Model file for the job. Use its own axes, mm. A direction names the side the tool comes from. Round coordinates to 2 decimals unless told otherwise and drop trailing zeros. Loops run counter-clockwise (first coordinate to the right, second up) from the corner with the lowest first, then second, coordinate; pieces in that order, holes last. Notation, with made-up numbers: M -14.75,27 L -3.75,27 A26 cw -3.75,65 Z; hole C 11.25,62.5 d11. An arc over 180 degrees is marked long. Use a Markdown table: item, result. Add a question column.
Q1. Cut at A-A (y = 0). Give the cut face in (x, z), plus the area to 3 significant figures.
Q2. Pin check, flat tips, straight feed: pin 1 (2.5 mm diameter, centred on y = 0, z = 2.5, fed in from +X); pin 2 (6.5 mm diameter, centred on x = 0, y = 0, fed in from +Z); pin 3 (1 mm diameter, centred on y = 6, z = 1.5, fed in from -X); pin 4 (3 mm diameter, centred on x = 3, z = 1.5, fed in from +Y). Stop position of each tip, or through.
Q3. Mould opens along Y. For faces 1 (the face through (-2.37, 4.495, 3.987)), 2 (the face through (3.81, -6.46, 2.46)), 3 (the face through (7.6, 2.5, 2.5)) say: +Y half, -Y half, draft (parallel to the pull), parting line (faces both ways), or undercut.
Q4. Probe line 1 (Z direction, x = 6.25, y = 0); line 2 (Y direction, x = 0, z = 1.95); line 3 (X direction, y = 0, z = 1.35). List the from-to ranges inside material, lowest first. Write a range as from..to.
Q5. Tool access for faces 4 (the face through (-5.947, 5.301, 2.465)), 5 (the face through (5, 0, 4)), 6 (the face through (8.071, -1, 1)), 7 (the face through (7.6, -2.5, 2.5)): list every direction of +Z, -Z, +X, -X, +Y, -Y with a clear straight run to the whole face (end or side of a thin tool).
Q6. Cut at C-C (x = 3.5). Give the cut face in (y, z).
Q7. Cut at D-D (x = 1.5). Give the cut face in (y, z).
Q8. Cut at B-B (z = 2.5). Give the cut face in (x, y), plus the area to 3 significant figures.
Autodesk Fusion 360 part; units mm, degrees
sketch "Boceto1" plane through (0, 0, 0) normal (0, 0, 1) x (1, 0, 0)
  circle A0 centre (0, 0) radius 2.5
  circle A1 centre (0, 0) radius 7.5
  line L0 (0, 2.5) -> (7.0711, 2.5)
  line L1 (0, -2.5) -> (7.0711, -2.5)
  line L2 (7.0711, 2.5) -> (7.0711, -2.5)
  line L3 (7.0711, 2.5) -> (8.0711, 2.5)
  line L4 (8.0711, 2.5) -> (8.0711, -2.5)
  line L5 (8.0711, -2.5) -> (7.0711, -2.5)
  line L6 (-6.2006, 5.7397) -> (-1.8705, 8.2397)
  line L7 (-5.7006, 4.8737) -> (-6.2006, 5.7397)
  line L8 (-1.8705, 8.2397) -> (-1.3705, 7.3737)
  line L9 (-1.8705, -8.2397) -> (-6.2006, -5.7397)
  line L10 (-1.3705, -7.3737) -> (-1.8705, -8.2397)
  line L11 (-6.2006, -5.7397) -> (-5.7006, -4.8737)
  dimension "d1" = 5
  dimension "d2" = 15
  dimension "d3" = 1
  dimension "d5" = 360
extrude "Extruir1" add sketch "Boceto1" along normal blind 5 contours A0 L0 L1 L2 | A0 A1 L0 L1 | A1 L3 L4 L5 | A1 L2 | A1 L6 L7 L8 | A1 L9 L10 L11
sketch "Boceto2" plane through (-4.0355, -6.9897, 0) normal (-0.5, -0.866, 0) x (0.866, -0.5, 0)
  line L0 (-2.5, 0) -> (2.5, 0)
  line L1 (2.5, 0) -> (2.5, 5)
  line L2 (2.5, 5) -> (-2.5, 5)
  line L3 (-2.5, 5) -> (-2.5, 0)
  line L4 (-2.5, 5) -> (2.5, 0)
  line L5 (2.5, 5) -> (-2.5, 0)
  circle A0 centre (0, 2.5) radius 1.5
  dimension "d8" = 3
sketch "Boceto3" plane through (8.0711, 0, 0) normal (1, 0, 0) x (0, 1, 0)
  line L0 (-2.5, 0) -> (2.5, 0)
  line L1 (2.5, 0) -> (2.5, 5)
  line L2 (2.5, 5) -> (-2.5, 5)
  line L3 (-2.5, 5) -> (-2.5, 0)
  line L4 (-2.5, 5) -> (2.5, 0)
  line L5 (2.5, 5) -> (-2.5, 0)
  circle A0 centre (0, 2.5) radius 1.5
  dimension "d9" = 3
sketch "Boceto4" plane through (-4.0355, 6.9897, 0) normal (-0.5, 0.866, 0) x (-0.866, -0.5, 0)
  line L0 (-2.5, 0) -> (2.5, 0)
  line L1 (2.5, 0) -> (2.5, 5)
  line L2 (2.5, 5) -> (-2.5, 5)
  line L3 (-2.5, 5) -> (-2.5, 0)
  line L4 (2.5, 5) -> (-2.5, 0)
  line L5 (-2.5, 5) -> (2.5, 0)
  circle A0 centre (0, 2.5) radius 1.5
  dimension "d10" = 3
extrude "Extruir2" cut sketch "Boceto4" against normal blind 8 contours L4 L5 A0 | L4 L5 A0 | L4 L5 A0 | L4 L5 A0
extrude "Extruir3" cut sketch "Boceto2" against normal blind 8 contours L4 L5 A0 | L4 L5 A0 | L4 L5 A0 | L4 L5 A0
extrude "Extruir4" cut sketch "Boceto3" against normal blind 8 contours L4 L5 A0 | L4 L5 A0 | L4 L5 A0 | L4 L5 A0
Checked values:
| question | item | result |
|---|---|---|
| 1 | outline | M -7.5,0 L -2.5,0 L -2.5,5 L -7.5,5 Z; M 2.5,0 L 8.07,0 L 8.07,1 L 2.5,1 Z; M 2.5,4 L 8.07,4 L 8.07,5 L 2.5,5 Z |
| 1 | area | 36.1 mm^2 |
| 2 | pin 1 | stops at x = -2.24 |
| 2 | pin 2 | stops at z = 5 |
| 2 | pin 3 | stops at x = -6.2 |
| 2 | pin 4 | stops at y = 7.35 |
| 3 | face 1 | undercut |
| 3 | face 2 | -Y half |
| 3 | face 3 | +Y half |
| 4 | line 1 | z = 0..1, 4..5 |
| 4 | line 2 | y = -7.5..-2.79, 2.79..7.5 |
| 4 | line 3 | x = -7.5..-2.5 |
| 5 | face 4 | +Z, -Z, -X |
| 5 | face 5 | +X |
| 5 | face 6 | +Z, -Z, +X, +Y, -Y |
| 5 | face 7 | +Z, -Z, +X, -Y |
| 6 | outline | M -6.63,0 L 6.63,0 L 6.63,5 L -6.63,5 Z; hole C 0,2.5 d3 |
| 7 | outline | M -7.35,0 L -2,0 L -2,5 L -7.35,5 Z; M 2,0 L 7.35,0 L 7.35,5 L 2,5 Z |
| 8 | outline | M -6.2,-5.74 L -5.33,-6.24 L -2.3,-0.98 A2.5 cw -2.3,0.98 L -5.33,6.24 L -6.2,5.74 L -5.7,4.87 A7.5 ccw -5.7,-4.87 Z; M -2.74,-7.74 L -1.87,-8.24 L -1.37,-7.37 A7.5 ccw 7.07,-2.5 L 8.07,-2.5 L 8.07,-1.5 L 2,-1.5 A2.5 cw 0.3,-2.48 Z; M -2.74,7.74 L 0.3,2.48 A2.5 cw 2,1.5 L 8.07,1.5 L 8.07,2.5 L 7.07,2.5 A7.5 ccw -1.37,7.37 L -1.87,8.24 Z |
| 8 | area | 116 mm^2 |
